from build123d import *

# Parameters (mm, degrees)
EXTRUDE_1_DEPTH     = 165
SKETCH_2_R          = 5
CUT_EXTRUDE_1_DEPTH = 10
SKETCH_3_R          = 5
CUT_EXTRUDE_2_DEPTH = 10
CUT_EXTRUDE_3_DEPTH = 66


with BuildPart() as part:
    # Эскиз1 → Вытянуть-Тонкостенный1 (new body)
    with BuildSketch(Plane(origin=(0, 0, 0), x_dir=(1, 0, 0), z_dir=(0, 1, 0))):
        Polygon((0, 65), (0, 0), (65, 0), (65, 4), (4, 4), (4, 65), align=None)
    extrude(amount=EXTRUDE_1_DEPTH)

    # Эскиз2 → Вырез-Вытянуть1 (cut)
    with BuildSketch(Plane.XY):
        with Locations((31, 120)):
            Circle(SKETCH_2_R)
        with Locations((31, 20)):
            Circle(SKETCH_2_R)
    extrude(amount=-CUT_EXTRUDE_1_DEPTH, mode=Mode.SUBTRACT)

    # Эскиз3 → Вырез-Вытянуть2 (cut)
    with BuildSketch(Plane.ZY):
        with Locations((-31, 120)):
            Circle(SKETCH_3_R)
        with Locations((-31, 20)):
            Circle(SKETCH_3_R)
        with Locations((-15, 155)):
            Circle(SKETCH_3_R)
        with Locations((-45, 155)):
            Circle(SKETCH_3_R)
    extrude(amount=-CUT_EXTRUDE_2_DEPTH, mode=Mode.SUBTRACT)

    # Эскиз4 → Вырез-Вытянуть3 (cut, through all)
    with BuildSketch(Plane.XY):
        Polygon((5, 165), (65, 125), (65, 165), align=None)
    extrude(amount=-CUT_EXTRUDE_3_DEPTH, mode=Mode.SUBTRACT)


solid = part.part
Here's how the part is built. I have some questions about the finished solid (model axes, mm). A direction names the side the tool comes from. Give positions to 0.01 mm unless a question says otherwise; leave off trailing zeros. Write each loop counter-clockwise with the first axis right and the second up, starting at its lowest first coordinate (ties: lowest second). Pieces come first, ordered by that corner, then holes. Notation, with made-up numbers: (-32.5, 54) -> (4.5, 54) arc R15 cw to (4.5, 61) -> close; hole circle Ø10 at (3, 26.25). An arc over 180 degrees is marked (long way). Use one line per item in the form item = value. Start each with the question number.
1. On a 3-axis mill with a long thin cutter (end or side, diameter ignored), from which of +Z, -Z, +X, -X, +Y, -Y can I reach the whole of each face in a straight line? I mean faces 1 (the face through (4, 81, -34)), 2 (the face through (2, 155, -50)). Say none if no direction works.
2. Imagine slicing it at B-B on z = -45. List the corners of the cut face in (x, y) for me, plus the area to 3 significant figures.
3. Imagine slicing it at C-C on x = 31. List the corners of the cut face in (y, z) for me.
4. Will these pins go through, and if not, where does the flat tip stop? pin 1 Ø16 at (y, z) = (155, -45) entering from +X; pin 2 Ø9 at (y, z) = (155, -15) entering from -X.
5. If I drill on L1, parallel to Y at x = 1, z = -31; L2, parallel to Y at x = 2.7, z = -45; L3, parallel to X at y = 108, z = -57, over which ranges is the centre line in solid material (lowest first)?
6. Thinking about a two-plate mould opening in Y: for faces 3 (the face through (3, 0, -18)), 4 (the face through (2, 17, -35)), 5 (the face through (0, 81, -33)), 6 (the face through (2, 165, -33)), which applies, +Y half, -Y half, draft (parallel to the pull), parting line (faces both ways), or undercut?
7. Imagine slicing it at A-A on y = 155. List the corners of the cut face in (x, z) for me, plus the area to 3 significant figures.
8. Imagine slicing it at D-D on x = 12.5. List the corners of the cut face in (y, z) for me, plus the area to 3 significant figures.
Entries:
q1.face_1 = -Z, +X, +Y, -Y
q1.face_2 = +X, -X
q2.outline = (0, 0) -> (4, 0) -> (4, 150) -> (0, 150) -> close; (0, 160) -> (4, 160) -> (4, 165) -> (0, 165) -> close
q2.area = 620 mm²
q3.outline = (0, -4) -> (15, -4) -> (15, 0) -> (0, 0) -> close; (25, -4) -> (115, -4) -> (115, 0) -> (25, 0) -> close; (125, -4) -> (147.67, -4) -> (147.67, 0) -> (125, 0) -> close
q4.pin_1 = 4
q4.pin_2 = through
q5.L1 = 0 to 15, 25 to 115, 125 to 165
q5.L2 = 0 to 150, 160 to 165
q5.L3 = 0 to 4
q6.face_3 = -Y half
q6.face_4 = undercut
q6.face_5 = draft
q6.face_6 = +Y half
q7.outline = (0, -65) -> (4, -65) -> (4, -50) -> (0, -50) -> close; (0, -40) -> (4, -40) -> (4, -20) -> (0, -20) -> close; (0, -10) -> (4, -10) -> (4, -4) -> (20, -4) -> (20, 0) -> (0, 0) -> close
q7.area = 244 mm²
q8.outline = (0, -4) -> (160, -4) -> (160, 0) -> (0, 0) -> close
q8.area = 640 mm²
